```python
from build123d import *

# Parameters (mm, degrees)
SKETCH1_W         = 50
SKETCH1_H         = 50
SKETCH1_R         = 1.5
SUPPORT_DEPTH     = 8
NORTH_START       = -25
SKETCH2_W         = 20
SKETCH2_H         = 5
NORTH_CUT_DEPTH   = 4
SOUTH_START       = 25
SKETCH2_2_W       = 20
SKETCH2_2_H       = 5
SOUTH_DOWEL_DEPTH = 4
WEST_START        = 25
SKETCH3_W         = 20
SKETCH3_H         = 5
WEST_DOWEL_DEPTH  = 4


with BuildPart() as part:
    # Sketch1 → Support (new body)
    with BuildSketch(Plane(origin=(0, 0, 0), x_dir=(1, 0, 0), z_dir=(0, 1, 0))):
        Rectangle(SKETCH1_W, SKETCH1_H)
        with Locations(Location((-21, -21, 0), (0, 0, 270))):
            Circle(SKETCH1_R, mode=Mode.SUBTRACT)
        with Locations(Location((21, -21, 0), (0, 0, 270))):
            Circle(SKETCH1_R, mode=Mode.SUBTRACT)
        with BuildLine():
            Line((-13.031373033, 17.5), (17.5, 17.5))
            Line((17.5, 17.5), (17.5, -17.5))
            Line((17.5, -17.5), (-17.5, -17.5))
            Line((-17.5, -17.5), (-17.5, 13.031373033))
            ThreePointArc((-17.5, 13.031373033), (-20, 14.354248689), (-21, 17))
            Line((-21, 17), (-22.130136986, 20.01369863))
            ThreePointArc((-22.130136986, 20.01369863), (-22.060660172, 22.060660172), (-20.01369863, 22.130136986))
            Line((-20.01369863, 22.130136986), (-17, 21))
            ThreePointArc((-17, 21), (-14.354248689, 20), (-13.031373033, 17.5))
        make_face(mode=Mode.SUBTRACT)
        with Locations(Location((21, 21, 0), (0, 0, 270))):
            Circle(SKETCH1_R, mode=Mode.SUBTRACT)
    extrude(amount=SUPPORT_DEPTH)

    # Sketch2 → North Cut (cut)
    with BuildSketch(Plane.XY.offset(NORTH_START)):
        with Locations((0, 4)):
            Rectangle(SKETCH2_W, SKETCH2_H)
    extrude(amount=NORTH_CUT_DEPTH, mode=Mode.SUBTRACT)

    # Sketch2<2> → South Dowel (add)
    with BuildSketch(Plane.XY.offset(SOUTH_START)):
        with Locations((0, 4)):
            Rectangle(SKETCH2_2_W, SKETCH2_2_H)
    extrude(amount=SOUTH_DOWEL_DEPTH)

    # Sketch3 → West Dowel (add)
    with BuildSketch(Plane(origin=(0, 0, 0), x_dir=(0, 0, -1), z_dir=(1, 0, 0)).offset(WEST_START)):
        with Locations((0, 4)):
            Rectangle(SKETCH3_W, SKETCH3_H)
    extrude(amount=WEST_DOWEL_DEPTH)


solid = part.part
```
Work out the finished part from the listing and answer in its coordinate system (mm). A direction names the side the tool comes from. Round coordinates to 2 decimals unless told otherwise and drop trailing zeros. Write each loop counter-clockwise with the first axis right and the second up, starting at its lowest first coordinate (ties: lowest second). Pieces come first, ordered by that corner, then holes. Notation, with made-up numbers: (22, 41) - (62, 41) arc R19 ccw to (62, 53) - close; hole circle Ø5 at (-34, 44). An arc over 180 degrees is marked (long way). Return JSON: item names as keys, results as strings. Group by question number.
Q1. The mould has two halves that part along X. Classify faces 6 (the flat face through (0, 7, -25)), 7 (the cylindrical face through (-19.99, 3.94, 19.89)), 8 (the flat face through (-17.5, 4, 2)): released by +X, released by -X, zero draft, split by the parting line, or undercut.
Q2. Each of these flat-tipped pins is pushed along its axis until it touches: pin 1 Ø1.2 at (y, z) = (5, 27) entering from +X; pin 2 Ø3 at (y, z) = (4.5, 27.5) entering from -X; pin 3 Ø1.2 at (x, z) = (27, -3) entering from +Y. Where does it stop, or does it pass through?
Q3. The part is cut by section A-A on y = 5.25. Write down the section's boundary in (x, z), then the cut area to 3 significant figures.
Q4. For faces 1 (the flat face through (27, 1.5, 0)), 2 (the flat face through (-21.56, 3.94, -18.49)), 3 (the flat face through (27, 6.5, 0)), 4 (the flat face through (27, 4, -10)), 5 (the flat face through (0, 6.5, -23)), determine the directions among +Z, -Z, +X, -X, +Y, -Y from which every point of the face is accessible in a straight line to the end or side of a thin tool.
Q5. Find the intervals of material crossed by L1, parallel to X at y = 5.5, z = 21; L2, parallel to X at y = 4, z = -1.5; L3, parallel to Z at x = 3, y = 2.25, in increasing order.
Q6. The part is cut by section D-D on x = -11.5. Write down the section's boundary in (y, z), then the cut area to 3 significant figures.
Q7. The part is cut by section C-C on z = 21. Write down the section's boundary in (x, y).
Q8. The part is cut by section B-B on x = 21. Write down the section's boundary in (y, z).
Solved:
{
 "1": {"face 6": "zero draft", "face 7": "undercut", "face 8": "undercut"},
 "2": {"pin 1": "x = 10", "pin 2": "x = -10", "pin 3": "y = 6.5"},
 "3": {"outline": "(-25, -25) - (-10, -25) - (-10, -21) - (10, -21) - (10, -25) - (25, -25) - (25, -10) - (29, -10) - (29, 10) - (25, 10) - (25, 25) - (10, 25) - (10, 29) - (-10, 29) - (-10, 25) - (-25, 25) - close; hole circle Ø3 at (-21, 21); hole (-22.13, -20.01) arc R1.5 ccw to (-20.01, -22.13) - (-17, -21) arc R4 ccw to (-13.03, -17.5) - (17.5, -17.5) - (17.5, 17.5) - (-17.5, 17.5) - (-17.5, -13.03) arc R4 ccw to (-21, -17) - close; hole circle Ø3 at (21, -21); hole circle Ø3 at (21, 21)", "area": "1,290 mm²"},
 "4": {"face 1": "+Z, -Z, +X, -Y", "face 2": "+Y, -Y", "face 3": "+Z, -Z, +X, +Y", "face 4": "-Z, +X, +Y, -Y", "face 5": "-Z"},
 "5": {"L1": "-25 to -22.5, -19.5 to 19.5, 22.5 to 25", "L2": "-25 to -17.5, 17.5 to 29", "L3": "-21 to -17.5, 17.5 to 29"},
 "6": {"outline": "(0, -25) - (8, -25) - (8, -17.5) - (0, -17.5) - close; (0, 17.5) - (8, 17.5) - (8, 25) - (0, 25) - close", "area": "120 mm²"},
 "7": {"outline": "(-25, 0) - (-22.5, 0) - (-22.5, 8) - (-25, 8) - close; (-19.5, 0) - (19.5, 0) - (19.5, 8) - (-19.5, 8) - close; (22.5, 0) - (25, 0) - (25, 8) - (22.5, 8) - close"},
 "8": {"outline": "(0, -25) - (8, -25) - (8, -22.5) - (0, -22.5) - close; (0, -19.5) - (8, -19.5) - (8, 19.5) - (0, 19.5) - close; (0, 22.5) - (8, 22.5) - (8, 25) - (0, 25) - close"}
}
